```python
from build123d import *

# Parameters (mm, degrees)
F0_W      = 57
F0_H      = 37
F0_W_2    = 47
F0_H_2    = 27
F1_DEPTH  = 1.2
F2_W      = 57
F2_H      = 37
F2_W_2    = 51
F2_H_2    = 31
F3_DEPTH  = 3
F4_W      = 57
F4_H      = 37
F4_W_2    = 54
F4_H_2    = 34
F5_DEPTH  = 40
F6_W      = 55.5
F6_H      = 5
F7_DEPTH  = 25
F9_D      = 4.2
F11_D     = 8
F11_DEPTH = 5


with BuildPart() as f1:
    # F0 (on Front) → F1 (new body)
    with BuildSketch(Plane.XZ):
        Rectangle(F0_W, F0_H)
        Rectangle(F0_W_2, F0_H_2, mode=Mode.SUBTRACT)
    extrude(amount=F1_DEPTH)

    # F2 (on face) → F3 (join)
    with BuildSketch(Plane.XZ.offset(1.2)):
        Rectangle(F2_W, F2_H)
        Rectangle(F2_W_2, F2_H_2, mode=Mode.SUBTRACT)
    extrude(amount=F3_DEPTH)

    # F4 (on face) → F5 (join)
    with BuildSketch(Plane(origin=(0, 0, 0), x_dir=(-1, 0, 0), z_dir=(0, 1, 0))):
        Rectangle(F4_W, F4_H)
        Rectangle(F4_W_2, F4_H_2, mode=Mode.SUBTRACT)
    extrude(amount=F5_DEPTH)

    # F6 (on face) → F7 (join)
    with BuildSketch(Plane.XY.offset(18.5)):
        with Locations((0, 10.8)):
            Rectangle(F6_W, F6_H)
    extrude(amount=F7_DEPTH)

    # F9 (through all)
    with Locations(Plane.XZ.offset(-8.3)):
        with Locations((-17.75, 31), (17.75, 31)):
            Hole(F9_D / 2)

    # F11
    with Locations(Plane(origin=(-28.5, 0, 0), x_dir=(0, -1, 0), z_dir=(-1, 0, 0))):
        with Locations((-32.028917, 0)):
            Hole(F11_D / 2, depth=F11_DEPTH)


solid = f1.part
```
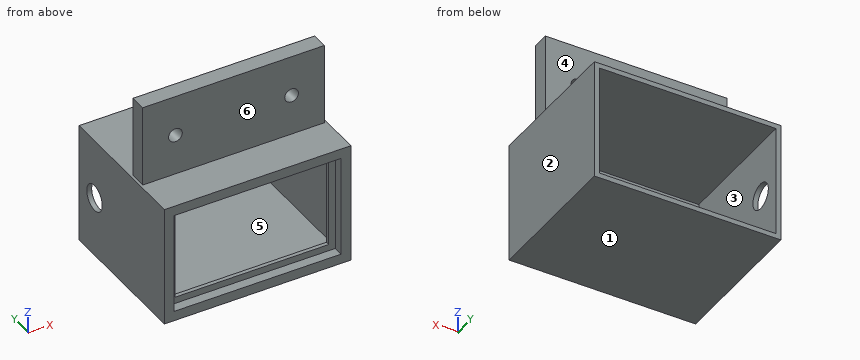
The model under review builds one solid part; all positions refer to its coordinate system, in mm. Face numbers are marked on the shaded views. A direction names the side the tool comes from. Give positions to 0.01 mm unless a question says otherwise; leave off trailing zeros. Write each loop counter-clockwise with the first axis right and the second up, starting at its lowest first coordinate (ties: lowest second). Pieces come first, ordered by that corner, then holes. Notation, with made-up numbers: M -2.75,-39.75 L 34.25,-39.75 A18 ccw 34.25,-13.75 Z; hole C 21,-2.5 d6. An arc over 180 degrees is marked long. Write each question's results on one line, items separated by ' | '. Start each with the question number.
1. For the marked faces 4, 5 and 6, list the 3-axis set-ups (+Z, -Z, +X, -X, +Y, -Y) from which the entire face can be reached by the end or side of a thin tool; tool diameter is ignored.
2. For probe 1 along Z at (x, y) = (17.75, 11.2); probe 2 along X at (y, z) = (17, 6); probe 3 along Z at (x, y) = (-5, 13.5), list the stretches that pass through material, from the lowest coordinate up. Write a range as [from, to].
3. Insertion check: pin 1 Ø1.5 at (x, z) = (-3.5, 24.5) entering from -Y; pin 2 Ø2.5 at (y, z) = (11, 25.5) entering from +X; pin 3 Ø9 at (y, z) = (32.03, 0) entering from -X; pin 4 Ø7.5 at (x, z) = (-10, 26) entering from +Y. Each pin has a flat end and moves straight along its axis. Give the tip position at first contact, or say it passes through.
4. We need section D-D (x = 17.75). Write out the cut boundary in (y, z), and give its area (3 significant figures).
5. We need section B-B (x = 0). Write out the cut boundary in (y, z), and give its area (3 significant figures).
6. Mouldability with a two-part tool opening along X and no side actions: class the marked faces 1, 2 and 3 as released by +X, released by -X, zero draft, split by the parting line, or undercut.
7. We need section A-A (z = 31). Write out the cut boundary in (x, y).
8. We need section C-C (y = 22.5). Write out the cut boundary in (x, z).
Results found:
1) face 4: +Z, +X, -X, +Y | face 5: +Y | face 6: +Z, +X, -X, -Y
2) probe 1: z = [-18.5, -17], [17, 28.9], [33.1, 43.5] | probe 2: x = [-28.5, -27], [27, 28.5] | probe 3: z = [-18.5, -17], [17, 18.5]
3) pin 1: stops at y = 8.3 | pin 2: stops at x = 27.75 | pin 3: stops at x = -28.5 | pin 4: stops at y = 13.3
4) outline: M -4.2,-18.5 L 40,-18.5 L 40,-17 L 0,-17 L 0,-13.5 L -1.2,-13.5 L -1.2,-15.5 L -4.2,-15.5 Z; M -4.2,15.5 L -1.2,15.5 L -1.2,13.5 L 0,13.5 L 0,17 L 40,17 L 40,18.5 L 13.3,18.5 L 13.3,28.9 L 8.3,28.9 L 8.3,18.5 L -4.2,18.5 Z; M 8.3,33.1 L 13.3,33.1 L 13.3,43.5 L 8.3,43.5 Z | area: 254 mm^2
5) outline: M -4.2,-18.5 L 40,-18.5 L 40,-17 L 0,-17 L 0,-13.5 L -1.2,-13.5 L -1.2,-15.5 L -4.2,-15.5 Z; M -4.2,15.5 L -1.2,15.5 L -1.2,13.5 L 0,13.5 L 0,17 L 40,17 L 40,18.5 L 13.3,18.5 L 13.3,43.5 L 8.3,43.5 L 8.3,18.5 L -4.2,18.5 Z | area: 275 mm^2
6) face 1: zero draft | face 2: released by +X | face 3: undercut
7) outline: M -27.75,8.3 L -19.85,8.3 L -19.85,13.3 L -27.75,13.3 Z; M -15.65,8.3 L 15.65,8.3 L 15.65,13.3 L -15.65,13.3 Z; M 19.85,8.3 L 27.75,8.3 L 27.75,13.3 L 19.85,13.3 Z
8) outline: M -28.5,-18.5 L 28.5,-18.5 L 28.5,18.5 L -28.5,18.5 Z; hole M -27,-17 L 27,-17 L 27,17 L -27,17 Z
